Can you work these out from the model? Positions are in its coordinate system, mm. Face numbers are marked on the shaded views. Round coordinates to 2 decimals unless told otherwise and drop trailing zeros. Order: outer loops, then holes, each group sorted by start corner. A loop starts at its lowest first (then second) coordinate and runs counter-clockwise, first axis right, second up. Notation, with made-up numbers: (51, 18.25) -> (63, 18.25) arc R24 cw to (63, 44.25) -> close; hole circle Ø11 at (44.25, -29). An arc over 180 degrees is marked (long way). One line per item, written item: value.
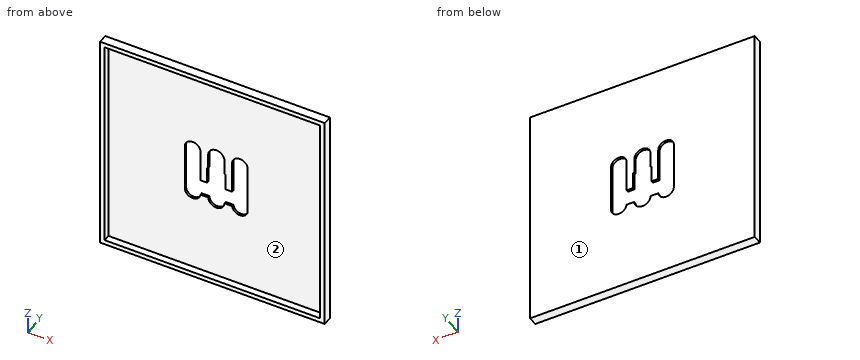
```python
from build123d import *

# Parameters (mm, degrees)
SKETCH1_W           = 100
SKETCH1_H           = 100
SKETCH1_W_2         = 96
SKETCH1_H_2         = 96
BOSS_EXTRUDE1_DEPTH = 3
SKETCH2_W           = 100
SKETCH2_H           = 100
BOSS_EXTRUDE2_DEPTH = 1
CUT_EXTRUDE1_DEPTH  = 1


with BuildPart() as part:
    # Sketch1 → Boss-Extrude1 (new body)
    with BuildSketch(Plane(origin=(0, 0, 0), x_dir=(1, 0, 0), z_dir=(0, 1, 0))):
        Rectangle(SKETCH1_W, SKETCH1_H)
        Rectangle(SKETCH1_W_2, SKETCH1_H_2, mode=Mode.SUBTRACT)
    extrude(amount=BOSS_EXTRUDE1_DEPTH)

    # Sketch2 → Boss-Extrude2 (add)
    with BuildSketch(Plane(origin=(0, 3, 0), x_dir=(1, 0, 0), z_dir=(0, 1, 0))):
        Rectangle(SKETCH2_W, SKETCH2_H)
    extrude(amount=BOSS_EXTRUDE2_DEPTH)

    # Sketch3 → Cut-Extrude1 (cut)
    with BuildSketch(Plane.XZ.offset(-3)):
        with BuildLine():
            Line((-7.034769829, -3.709104883), (-7.034769829, 10.517384915))
            ThreePointArc((-7.034769829, 10.517384915), (-10.517384915, 14), (-14, 10.517384915))
            Line((-14, 10.517384915), (-14, -10.517384915))
            ThreePointArc((-14, -10.517384915), (-10.687570013, -13.995839293), (-7.051402714, -10.857348469))
            Line((-7.051402714, -10.857348469), (-3.591574507, -10.857348469))
            ThreePointArc((-3.591574507, -10.857348469), (0, -14.448922976), (3.591574507, -10.857348469))
            Line((3.591574507, -10.857348469), (7.051402714, -10.857348469))
            ThreePointArc((7.051402714, -10.857348469), (10.687570013, -13.995839293), (14, -10.517384915))
            Line((14, -10.517384915), (14, 10.517384915))
            ThreePointArc((14, 10.517384915), (10.517384915, 14), (7.034769829, 10.517384915))
            Line((7.034769829, 10.517384915), (7.034769829, -3.709104883))
            Line((7.034769829, -3.709104883), (4.104776873, -3.709104883))
            Line((4.104776873, -3.709104883), (4.104776873, 3.709104883))
            Line((4.104776873, 3.709104883), (3.591574507, 3.709104883))
            Line((3.591574507, 3.709104883), (3.591574507, 10.517384915))
            ThreePointArc((3.591574507, 10.517384915), (0, 14.108959421), (-3.591574507, 10.517384915))
            Line((-3.591574507, 10.517384915), (-3.591574507, 3.709104883))
            Line((-3.591574507, 3.709104883), (-4.104776873, 3.709104883))
            Line((-4.104776873, 3.709104883), (-4.104776873, -3.709104883))
            Line((-4.104776873, -3.709104883), (-7.034769829, -3.709104883))
        make_face()
    extrude(amount=-CUT_EXTRUDE1_DEPTH, mode=Mode.SUBTRACT)


solid = part.part
```
Q1. I want a section at D-D on x = 31. List the corners of the cut face in (y, z) for me.
Answers below:
outline: (0, -50) -> (4, -50) -> (4, 50) -> (0, 50) -> (0, 48) -> (3, 48) -> (3, -48) -> (0, -48) -> close
Q2. Please list where these lines run through material, in increasing order: line 1 along X through (y, z) = (3.45, 7.5); line 2 along X through (y, z) = (1.9, 23).
Answers below:
line 1: -50 to -14, -7.03 to -3.59, 3.59 to 7.03, 14 to 50
line 2: -50 to -48, 48 to 50
Q3. I want a section at A-A on y = 2.05. List the corners of the cut face in (x, z) for me, plus the area to 3 significant figures.
Answers below:
outline: (-50, -50) -> (50, -50) -> (50, 50) -> (-50, 50) -> close; hole (-48, -48) -> (48, -48) -> (48, 48) -> (-48, 48) -> close
area: 784 mm^2
Q4. I want a section at B-B on x = 0. List the corners of the cut face in (y, z) for me, plus the area to 3 significant figures.
Answers below:
outline: (0, -50) -> (4, -50) -> (4, -14.45) -> (3, -14.45) -> (3, -48) -> (0, -48) -> close; (0, 48) -> (3, 48) -> (3, 14.11) -> (4, 14.11) -> (4, 50) -> (0, 50) -> close
area: 83.4 mm^2
Q5. I want a section at C-C on z = -17. List the corners of the cut face in (x, y) for me, plus the area to 3 significant figures.
Answers below:
outline: (-50, 0) -> (-48, 0) -> (-48, 3) -> (48, 3) -> (48, 0) -> (50, 0) -> (50, 4) -> (-50, 4) -> close
area: 112 mm^2
Q6. Will this pin go through, and if not, where does the flat tip stop? pin 1 Ø3 at (x, z) = (-22, -30) entering from -Y.
Answers below:
pin 1: y = 3
Q7. We'd pull the mould along Z, two halves only. Please class the marked faces 1 and 2: released by +Z, released by -Z, zero draft, split by the parting line, or undercut.
Answers below:
face 1: zero draft
face 2: undercut
